from build123d import *

# Parameters (mm, degrees)
SKETCH1_R           = 20.6375
SKETCH1_R_2         = 14.2875
SKETCH1_R_3         = 4.7625
SKETCH1_R_4         = 2.4892
BOSS_EXTRUDE1_DEPTH = 3.175


with BuildPart() as part:
    # Sketch1 → Boss-Extrude1 (new, symmetric)
    # profile 1 of 7: a face of its own
    with BuildSketch(Plane.XY):
        Circle(SKETCH1_R)
        Circle(SKETCH1_R_2, mode=Mode.SUBTRACT)
    # profile 2 of 7: a face of its own
    with BuildSketch(Plane.XY):
        with BuildLine():
            ThreePointArc((4.7625, 41.275), (-0.207737332, 36.517032845), (-4.74437725, 41.690079225))
            Line((-4.74437725, 41.690079225), (-6.68354577, 19.525281616))
            ThreePointArc((-6.68354577, 19.525281616), (0, 20.6375), (6.68354577, 19.525281616))
            Line((6.68354577, 19.525281616), (4.74437725, 41.690079225))
            ThreePointArc((4.74437725, 41.690079225), (4.757967155, 41.482737332), (4.7625, 41.275))
        make_face()
    # profile 3 of 7: a face of its own
    with BuildSketch(Plane.XY):
        with BuildLine():
            Line((34.986080435, -23.163462544), (19.253333892, -7.430716001))
            ThreePointArc((19.253333892, -7.430716001), (15.809242195, -13.265529295), (10.661133073, -17.670502196))
            Line((10.661133073, -17.670502196), (28.886826612, -30.432270201))
            ThreePointArc((28.886826612, -30.432270201), (27.970197729, -23.469782599), (34.986080435, -23.163462544))
        make_face()
    # profile 4 of 7: a face of its own
    with BuildSketch(Plane.XY):
        with BuildLine():
            ThreePointArc((-10.661133073, -17.670502196), (-15.809242195, -13.265529295), (-19.253333892, -7.430716001))
            Line((-19.253333892, -7.430716001), (-34.986080435, -23.163462544))
            ThreePointArc((-34.986080435, -23.163462544), (-29.795954543, -22.131082316), (-26.85598439, -26.53105859))
            ThreePointArc((-26.85598439, -26.53105859), (-27.394095297, -28.73013636), (-28.886826612, -30.432270201))
            Line((-28.886826612, -30.432270201), (-10.661133073, -17.670502196))
        make_face()
    # profile 5 of 7: a face of its own
    with BuildSketch(Plane.XY):
        with Locations((-31.61848439, -26.53105859)):
            Circle(SKETCH1_R_3)
        with Locations((-31.61848439, -26.53105859)):
            Circle(SKETCH1_R_4, mode=Mode.SUBTRACT)
    # profile 6 of 7: a face of its own
    with BuildSketch(Plane.XY):
        with Locations((0, 41.275)):
            Circle(SKETCH1_R_3)
        with Locations((0, 41.275)):
            Circle(SKETCH1_R_4, mode=Mode.SUBTRACT)
    # profile 7 of 7: a face of its own
    with BuildSketch(Plane.XY):
        with Locations((31.61848439, -26.53105859)):
            Circle(SKETCH1_R_3)
        with Locations((31.61848439, -26.53105859)):
            Circle(SKETCH1_R_4, mode=Mode.SUBTRACT)
    extrude(amount=BOSS_EXTRUDE1_DEPTH, both=True)


solid = part.part
Input: part model. Units: mm. Frame: model coordinates. Coordinates: 2 decimals unless noted, no trailing zeros. Loops run counter-clockwise (first coordinate to the right, second up) from the corner with the lowest first, then second, coordinate; pieces in that order, holes last.
Q1. Material intervals for line 1 (Y direction, x = 0, z = 2.2); line 2 (X direction, y = -19, z = -0.25); line 3 (Y direction, x = -1, z = 1), sorted ascending.
Q2. Draft query along Y for faces 1 (the face through (11, -10, -3.175)), 2 (the face through (35.2, -29.67, 0.04)), 3 (the face through (18.8, 8.51, 0.04)). Return one class per face: +Y half, -Y half, draft (parallel to the pull), parting line (faces both ways), or undercut.
Q3. Cut plane A-A (y = 0). Output: boundary loops of the cut face in (x, z) (1 decimal).
Q4. Cut plane C-C (z = -2.25). Output: boundary loops of the cut face in (x, y) (1 decimal).
Q5. Cut plane D-D (y = 10). Output: boundary loops of the cut face in (x, z) (3 decimals).
Q6. Cut plane B-B (x = 0). Output: boundary loops of the cut face in (y, z) (1 decimal), then the cut area to 3 significant figures.
Q7. Contact query for flat-ended pins moving along their axis: pin 1 (4 mm diameter, centred on x = 31.62, y = -26.53, fed in from -Z); pin 2 (1 mm diameter, centred on y = -17, z = 0, fed in from -X). Output: stop coordinate, or through.
Working result:
1. line 1: y = -20.64 to -14.29, 14.29 to 38.79, 43.76 to 46.04
1. line 2: x = -30.82 to -12.56, -8.06 to 8.06, 12.56 to 30.82
1. line 3: y = -20.61 to -14.25, 14.25 to 39, 43.55 to 45.93
2. face 1: draft
2. face 2: parting line
2. face 3: undercut
3. outline: (-20.6, -3.2) - (-14.3, -3.2) - (-14.3, 3.2) - (-20.6, 3.2) - close; (14.3, -3.2) - (20.6, -3.2) - (20.6, 3.2) - (14.3, 3.2) - close
4. outline: (-35, -23.2) arc R4.8 ccw to (-28.9, -30.4) - (-10.7, -17.7) arc R20.6 ccw to (10.7, -17.7) - (28.9, -30.4) arc R4.8 ccw to (35, -23.2) - (19.3, -7.4) arc R20.6 ccw to (6.7, 19.5) - (4.7, 41.7) arc R4.8 ccw to (-4.7, 41.7) - (-6.7, 19.5) arc R20.6 ccw to (-19.3, -7.4) - close; hole circle Ø5 at (-31.6, -26.5); hole circle Ø28.6 at (0, 0); hole circle Ø5 at (0, 41.3); hole circle Ø5 at (31.6, -26.5)
5. outline: (-18.053, -3.175) - (-10.205, -3.175) - (-10.205, 3.175) - (-18.053, 3.175) - close; (10.205, -3.175) - (18.053, -3.175) - (18.053, 3.175) - (10.205, 3.175) - close
6. outline: (-20.6, -3.2) - (-14.3, -3.2) - (-14.3, 3.2) - (-20.6, 3.2) - close; (14.3, -3.2) - (38.8, -3.2) - (38.8, 3.2) - (14.3, 3.2) - close; (43.8, -3.2) - (46, -3.2) - (46, 3.2) - (43.8, 3.2) - close
6. area: 210 mm2
7. pin 1: passes through
7. pin 2: stops at x = -29.32
